from build123d import *

# Parameters (mm, degrees)
BOSS_EXTRUDE1_DEPTH = 3.175
SKETCH2_R           = 2.4638
CUT_EXTRUDE1_DEPTH  = 6.35
SKETCH3_R           = 2.159
CUT_EXTRUDE2_DEPTH  = 6.35
SKETCH4_R           = 2.2225
SKETCH4_R_2         = 2.286
CUT_EXTRUDE3_DEPTH  = 351.937720963
SKETCH5_R           = 1.651
CUT_EXTRUDE4_DEPTH  = 351.937720963
SKETCH6_R           = 2.032
SKETCH6_R_2         = 2.159
SKETCH6_R_3         = 1.397
SKETCH6_R_4         = 1.5499969
CUT_EXTRUDE5_DEPTH  = 351.937720963
SKETCH7_R           = 2.159
CUT_EXTRUDE6_DEPTH  = 351.937720963
CUT_EXTRUDE8_DEPTH  = 351.937720963


with BuildPart() as part:
    # Sketch1 → Boss-Extrude1 (new body)
    with BuildSketch(Plane(origin=(0, 0, 0), x_dir=(1, 0, 0), z_dir=(0, 1, 0))):
        Polygon((-25.845025354, 51.656360067), (-61.766049839, 15.735335583), (-61.766049839, -217.222615449), (-25.845025354, -253.143639933), (207.112925677, -253.143639933), (243.033950161, -217.222615449), (243.033950161, 15.735335583), (207.112925677, 51.656360067), align=None)
    extrude(amount=BOSS_EXTRUDE1_DEPTH)

    # Sketch2 → Cut-Extrude1 (cut)
    with BuildSketch(Plane(origin=(0, 3.175, 0), x_dir=(1, 0, 0), z_dir=(0, 1, 0))):
        with Locations(Location((-17.872380726, 30.213331256, 0), (0, 0, 270))):
            Circle(SKETCH2_R)
        with Locations(Location((0.640891541, 11.70005899, 0), (0, 0, 270))):
            Circle(SKETCH2_R)
        with Locations(Location((-22.362508786, -10.197821288, 0), (0, 0, 270))):
            Circle(SKETCH2_R)
        with Locations(Location((-40.323021028, 7.762690954, 0), (0, 0, 270))):
            Circle(SKETCH2_R)
        with Locations(Location((203.630409109, -10.197821288, 0), (0, 0, 270))):
            Circle(SKETCH2_R)
        with Locations(Location((221.590921351, 7.762690954, 0), (0, 0, 270))):
            Circle(SKETCH2_R)
        with Locations(Location((180.627008782, 11.70005899, 0), (0, 0, 270))):
            Circle(SKETCH2_R)
        with Locations(Location((199.140281048, 30.213331256, 0), (0, 0, 270))):
            Circle(SKETCH2_R)
        with Locations(Location((-22.362508786, -191.289458578, 0), (0, 0, 270))):
            Circle(SKETCH2_R)
        with Locations(Location((-40.323021028, -209.24997082, 0), (0, 0, 270))):
            Circle(SKETCH2_R)
        with Locations(Location((-17.872380726, -231.700611123, 0), (0, 0, 270))):
            Circle(SKETCH2_R)
        with Locations(Location((0.640891541, -213.187338857, 0), (0, 0, 270))):
            Circle(SKETCH2_R)
        with Locations(Location((221.590921351, -209.24997082, 0), (0, 0, 270))):
            Circle(SKETCH2_R)
        with Locations(Location((199.140281048, -231.700611123, 0), (0, 0, 270))):
            Circle(SKETCH2_R)
        with Locations(Location((180.627008782, -213.187338857, 0), (0, 0, 270))):
            Circle(SKETCH2_R)
        with Locations(Location((203.630409109, -191.289458578, 0), (0, 0, 270))):
            Circle(SKETCH2_R)
    extrude(amount=-CUT_EXTRUDE1_DEPTH, mode=Mode.SUBTRACT)

    # Sketch3 → Cut-Extrude2 (cut)
    with BuildSketch(Plane(origin=(0, 3.175, 0), x_dir=(1, 0, 0), z_dir=(0, 1, 0))):
        with Locations(Location((73.488950161, -58.198639933, 0), (0, 0, 270))):
            Circle(SKETCH3_R)
        with Locations(Location((107.778950161, -58.198639933, 0), (0, 0, 270))):
            Circle(SKETCH3_R)
        with Locations(Location((73.488950161, -143.288639933, 0), (0, 0, 270))):
            Circle(SKETCH3_R)
        with Locations(Location((107.778950161, -143.288639933, 0), (0, 0, 270))):
            Circle(SKETCH3_R)
    extrude(amount=-CUT_EXTRUDE2_DEPTH, mode=Mode.SUBTRACT)

    # Sketch4 → Cut-Extrude3 (cut, through all)
    with BuildSketch(Plane(origin=(0, 3.175, 0), x_dir=(1, 0, 0), z_dir=(0, 1, 0))):
        with Locations(Location((42.754950161, 26.256360067, 0), (0, 0, 270))):
            Circle(SKETCH4_R)
        with Locations(Location((138.512950161, 26.256360067, 0), (0, 0, 270))):
            Circle(SKETCH4_R)
        with Locations(Location((42.754950161, -15.653639933, 0), (0, 0, 270))):
            Circle(SKETCH4_R)
        with Locations(Location((138.512950161, -15.653639933, 0), (0, 0, 270))):
            Circle(SKETCH4_R)
        with Locations(Location((138.512950161, -185.833639933, 0), (0, 0, 90))):
            Circle(SKETCH4_R)
        with Locations(Location((42.754950161, -185.833639933, 0), (0, 0, 90))):
            Circle(SKETCH4_R)
        with Locations(Location((138.512950161, -227.743639933, 0), (0, 0, 90))):
            Circle(SKETCH4_R)
        with Locations(Location((42.754950161, -227.743639933, 0), (0, 0, 90))):
            Circle(SKETCH4_R)
        with Locations(Location((69.678950161, -68.993639933, 0), (0, 0, 270))):
            Circle(SKETCH4_R_2)
        with Locations(Location((111.588950161, -68.993639933, 0), (0, 0, 270))):
            Circle(SKETCH4_R_2)
        with Locations(Location((69.678950161, -164.751639933, 0), (0, 0, 270))):
            Circle(SKETCH4_R_2)
        with Locations(Location((111.588950161, -164.751639933, 0), (0, 0, 270))):
            Circle(SKETCH4_R_2)
    extrude(amount=-CUT_EXTRUDE3_DEPTH, mode=Mode.SUBTRACT)

    # Sketch5 → Cut-Extrude4 (cut, through all)
    with BuildSketch(Plane(origin=(0, 3.175, 0), x_dir=(1, 0, 0), z_dir=(0, 1, 0))):
        with Locations(Location((-51.606049839, -84.741639933, 0), (0, 0, 270))):
            Circle(SKETCH5_R)
        with Locations(Location((-40.176049839, -84.741639933, 0), (0, 0, 270))):
            Circle(SKETCH5_R)
        with Locations(Location((-40.176049839, -116.745639933, 0), (0, 0, 90))):
            Circle(SKETCH5_R)
        with Locations(Location((-51.606049839, -116.745639933, 0), (0, 0, 90))):
            Circle(SKETCH5_R)
    extrude(amount=-CUT_EXTRUDE4_DEPTH, mode=Mode.SUBTRACT)

    # Sketch6 → Cut-Extrude5 (cut, through all)
    with BuildSketch(Plane(origin=(0, 3.175, 0), x_dir=(1, 0, 0), z_dir=(0, 1, 0))):
        with Locations(Location((101.301950161, -22.003639933, 0), (0, 0, 270))):
            Circle(SKETCH6_R)
        with Locations(Location((101.301950161, -50.959639933, 0), (0, 0, 270))):
            Circle(SKETCH6_R)
        with Locations(Location((128.733950161, -50.959639933, 0), (0, 0, 270))):
            Circle(SKETCH6_R)
        with Locations(Location((128.733950161, -22.003639933, 0), (0, 0, 270))):
            Circle(SKETCH6_R)
        with Locations(Location((57.613950161, 19.906360067, 0), (0, 0, 270))):
            Circle(SKETCH6_R_2)
        with Locations(Location((57.613950161, -4.223639933, 0), (0, 0, 270))):
            Circle(SKETCH6_R_2)
        with Locations(Location((123.653950161, -4.223639933, 0), (0, 0, 90))):
            Circle(SKETCH6_R_2)
        with Locations(Location((123.653950161, 19.906360067, 0), (0, 0, 90))):
            Circle(SKETCH6_R_2)
        with Locations(Location((75.647950161, -192.691639933, 0), (0, 0, 270))):
            Circle(SKETCH6_R_3)
        with Locations(Location((75.647950161, -222.663639933, 0), (0, 0, 270))):
            Circle(SKETCH6_R_3)
        with Locations(Location((105.619950161, -222.663639933, 0), (0, 0, 90))):
            Circle(SKETCH6_R_3)
        with Locations(Location((105.619950161, -192.691639933, 0), (0, 0, 90))):
            Circle(SKETCH6_R_3)
        with Locations(Location((52.533950161, -18.193639933, 0), (0, 0, 270))):
            Circle(SKETCH6_R_4)
        with Locations(Location((52.533950161, -48.593629933, 0), (0, 0, 270))):
            Circle(SKETCH6_R_4)
        with Locations(Location((76.533952961, -18.193639933, 0), (0, 0, 270))):
            Circle(SKETCH6_R_4)
        with Locations(Location((76.533952961, -48.593629933, 0), (0, 0, 270))):
            Circle(SKETCH6_R_4)
    extrude(amount=-CUT_EXTRUDE5_DEPTH, mode=Mode.SUBTRACT)

    # Sketch7 → Cut-Extrude6 (cut, through all)
    with BuildSketch(Plane(origin=(0, 3.175, 0), x_dir=(1, 0, 0), z_dir=(0, 1, 0))):
        with Locations(Location((65.233950161, 40.226360067, 0), (0, 0, 270))):
            Circle(SKETCH7_R)
        with Locations(Location((14.433950161, 40.226360067, 0), (0, 0, 270))):
            Circle(SKETCH7_R)
        with Locations(Location((-50.336049839, -75.343639933, 0), (0, 0, 270))):
            Circle(SKETCH7_R)
        with Locations(Location((-50.336049839, -24.543639933, 0), (0, 0, 270))):
            Circle(SKETCH7_R)
        with Locations(Location((231.603950161, -24.543639933, 0), (0, 0, 90))):
            Circle(SKETCH7_R)
        with Locations(Location((231.603950161, -75.343639933, 0), (0, 0, 90))):
            Circle(SKETCH7_R)
        with Locations(Location((166.833950161, 40.226360067, 0), (0, 0, 90))):
            Circle(SKETCH7_R)
        with Locations(Location((116.033950161, 40.226360067, 0), (0, 0, 90))):
            Circle(SKETCH7_R)
        with Locations(Location((116.033950161, -241.713639933, 0), (0, 0, 270))):
            Circle(SKETCH7_R)
        with Locations(Location((166.833950161, -241.713639933, 0), (0, 0, 270))):
            Circle(SKETCH7_R)
        with Locations(Location((231.603950161, -126.143639933, 0), (0, 0, 270))):
            Circle(SKETCH7_R)
        with Locations(Location((231.603950161, -176.943639933, 0), (0, 0, 270))):
            Circle(SKETCH7_R)
        with Locations(Location((-50.336049839, -176.943639933, 0), (0, 0, 90))):
            Circle(SKETCH7_R)
        with Locations(Location((-50.336049839, -126.143639933, 0), (0, 0, 90))):
            Circle(SKETCH7_R)
        with Locations(Location((14.433950161, -241.713639933, 0), (0, 0, 90))):
            Circle(SKETCH7_R)
        with Locations(Location((65.233950161, -241.713639933, 0), (0, 0, 90))):
            Circle(SKETCH7_R)
    extrude(amount=-CUT_EXTRUDE6_DEPTH, mode=Mode.SUBTRACT)

    # Sketch8 → Cut-Extrude8 (cut, through all)
    with BuildSketch(Plane(origin=(0, 3.175, 0), x_dir=(1, 0, 0), z_dir=(0, 1, 0))):
        with BuildLine():
            Line((-23.031049839, -68.993639933), (-23.031049839, -132.493639933))
            ThreePointArc((-23.031049839, -132.493639933), (-26.206049839, -135.668639933), (-29.381049839, -132.493639933))
            Line((-29.381049839, -132.493639933), (-29.381049839, -68.993639933))
            ThreePointArc((-29.381049839, -68.993639933), (-26.206049839, -65.818639933), (-23.031049839, -68.993639933))
        make_face()
        with BuildLine():
            Line((34.118950161, -68.993639933), (34.118950161, -132.493639933))
            ThreePointArc((34.118950161, -132.493639933), (30.943950161, -135.668639933), (27.768950161, -132.493639933))
            Line((27.768950161, -132.493639933), (27.768950161, -68.993639933))
            ThreePointArc((27.768950161, -68.993639933), (30.943950161, -65.818639933), (34.118950161, -68.993639933))
        make_face()
        with BuildLine():
            Line((204.298950161, -68.993639933), (204.298950161, -132.493639933))
            ThreePointArc((204.298950161, -132.493639933), (207.473950161, -135.668639933), (210.648950161, -132.493639933))
            Line((210.648950161, -132.493639933), (210.648950161, -68.993639933))
            ThreePointArc((210.648950161, -68.993639933), (207.473950161, -65.818639933), (204.298950161, -68.993639933))
        make_face()
        with BuildLine():
            Line((147.148950161, -68.993639933), (147.148950161, -132.493639933))
            ThreePointArc((147.148950161, -132.493639933), (150.323950161, -135.668639933), (153.498950161, -132.493639933))
            Line((153.498950161, -132.493639933), (153.498950161, -68.993639933))
            ThreePointArc((153.498950161, -68.993639933), (150.323950161, -65.818639933), (147.148950161, -68.993639933))
        make_face()
    extrude(amount=-CUT_EXTRUDE8_DEPTH, mode=Mode.SUBTRACT)


solid = part.part
Here's how the part is built. I have some questions about the finished solid (model axes, mm). Give positions to 0.01 mm unless a question says otherwise; leave off trailing zeros. Order: outer loops, then holes, each group sorted by start corner. A loop starts at its lowest first (then second) coordinate and runs counter-clockwise, first axis right, second up. Notation, with made-up numbers: (4.25, 66) -> (48.25, 66) arc R25 cw to (48.25, 87) -> close; hole circle Ø8 at (79.25, 0). An arc over 180 degrees is marked (long way). Use a Markdown table: item, result. Add a question column.
Item 1: Imagine slicing it at B-B on y = 1.5. Give the number of separate pieces and of enclosed holes in the cut face, plus the area to 3 significant figures.
Item 2: I need wall thicknesses on line 1 (Z direction, x = 167, y = 0.95); line 2 (X direction, y = 1.75, z = 25); line 3 (Z direction, x = 111.5, y = 0.95). Which ranges of each line are inside material? Lowest first, please.
Item 3: Imagine slicing it at A-A on z = 95. Please give me the cut outline in (x, y) (3 decimals), plus the area to 3 significant figures.
Item 4: Will this pin go through, and if not, where does the flat tip stop? pin 1 (4 mm diameter, centred on x = 231.6, z = 75.34, fed in from +Y).
Data:
| question | item | result |
|---|---|---|
| 1 | separate pieces | 1 |
| 1 | enclosed holes | 72 |
| 1 | area | 87,600 mm² |
| 2 | line 1 | z = -51.66 to -42.38, -38.07 to 239.56, 243.87 to 253.14 |
| 2 | line 2 | x = -61.77 to -52.45, -48.23 to 229.49, 233.71 to 243.03 |
| 2 | line 3 | z = -51.66 to 66.71, 71.28 to 162.47, 167.04 to 253.14 |
| 3 | outline | (-61.766, 0) -> (-29.381, 0) -> (-29.381, 3.175) -> (-61.766, 3.175) -> close; (-23.031, 0) -> (27.769, 0) -> (27.769, 3.175) -> (-23.031, 3.175) -> close; (34.119, 0) -> (147.149, 0) -> (147.149, 3.175) -> (34.119, 3.175) -> close; (153.499, 0) -> (204.299, 0) -> (204.299, 3.175) -> (153.499, 3.175) -> close; (210.649, 0) -> (243.034, 0) -> (243.034, 3.175) -> (210.649, 3.175) -> close |
| 3 | area | 887 mm² |
| 4 | pin 1 | passes through |
